Geometry check sheet. Reference: the model listing, model coordinates, mm. Face numbers are marked on the shaded views. A direction names the side the tool comes from. Round coordinates to 2 decimals unless told otherwise and drop trailing zeros. Loops run counter-clockwise (first coordinate to the right, second up) from the corner with the lowest first, then second, coordinate; pieces in that order, holes last. Notation, with made-up numbers: M -35,48 L -1,48 A35 cw -1,83 Z; hole C -23,-12 d10. An arc over 180 degrees is marked long. Write item = value, one per line.
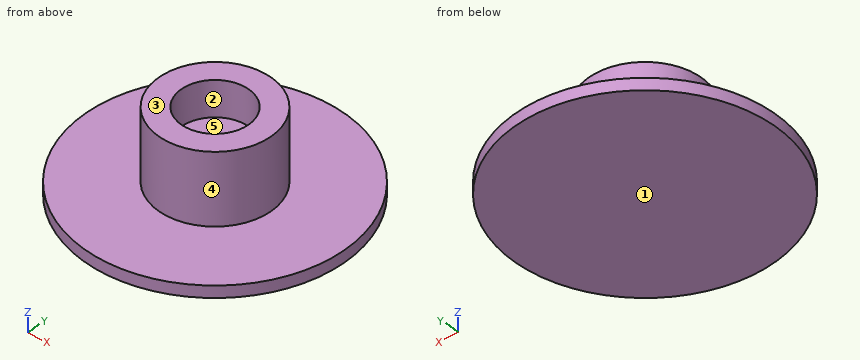
from build123d import *

# Parameters (mm, degrees)
F0_R     = 4.7625
F0_R_2   = 2.613606
F1_DEPTH = 7
F0_R_3   = 11
F2_DEPTH = 1
F3_R     = 2.8575
F4_DEPTH = 3


with BuildPart() as f1:
    # F0 (on Top) → F1 (new body)
    with BuildSketch(Plane.XY):
        Circle(F0_R)
        Circle(F0_R_2, mode=Mode.SUBTRACT)
        Circle(F0_R_2)
    extrude(amount=F1_DEPTH)

    # F0 (on Top) → F2 (join)
    with BuildSketch(Plane.XY):
        Circle(F0_R_3)
        Circle(F0_R, mode=Mode.SUBTRACT)
    extrude(amount=F2_DEPTH)

    # F3 (on face) → F4 (cut)
    with BuildSketch(Plane.XY.offset(7)):
        Circle(F3_R)
    extrude(amount=-F4_DEPTH, mode=Mode.SUBTRACT)


solid = f1.part
(1) Sectioned sample at C-C on z = 5.75. Record the cut outline in (x, y) (1 decimal).
Result set:
outline = C 0,0 d9.5; hole C 0,0 d5.7
(2) Tool access check on the marked faces 1 and 2. Record the directions out of +Z, -Z, +X, -X, +Y, -Y that give a thin tool (end or side, any length) a straight path to the whole face; none if there is none.
Result set:
face_1 = -Z, +X, -X, +Y, -Y
face_2 = +Z
(3) Sectioned sample at A-A on y = 0. Record the cut outline in (x, z).
Result set:
outline = M -11,0 L 11,0 L 11,1 L 4.76,1 L 4.76,7 L 2.86,7 L 2.86,4 L -2.86,4 L -2.86,7 L -4.76,7 L -4.76,1 L -11,1 Z
(4) Depth check by flat-ended pin: pin 1 Ø4 at (x, z) = (-8, 2.5) entering from +Y; pin 2 Ø1.7 at (x, y) = (0.5, 0.5) entering from +Z; pin 3 Ø6 at (x, y) = (-8.5, -2) entering from +Z. Enter the tip coordinate at first touch or a pass-through.
Result set:
pin_1 = 8.74
pin_2 = 4
pin_3 = 1
(5) Material ranges on line 1 along Y through (x, z) = (0, 5.7); line 2 along Z through (x, y) = (-3.5, -5.75); line 3 along X through (y, z) = (0.5, 6.5), recorded low to high. Write a range as from..to.
Result set:
line_1 = -4.76..-2.86, 2.86..4.76
line_2 = 0..1
line_3 = -4.74..-2.81, 2.81..4.74
(6) Sectioned sample at D-D on z = 1.5. Record the cut outline in (x, y) (1 decimal).
Result set:
outline = C 0,0 d9.5
(7) Release check for a two-part mould opening along Y. For the marked faces 3, 4 and 5 record: released by +Y, released by -Y, zero draft, split by the parting line, or undercut.
Result set:
face_3 = zero draft
face_4 = split by the parting line
face_5 = undercut
